For this review, use the dimensioned drawing (mm, ordinates from the lowest corner) and the shaded views. A direction names the side the tool comes from. Give positions to 0.01 mm unless a question says otherwise; leave off trailing zeros. Write each loop counter-clockwise with the first axis right and the second up, starting at its lowest first coordinate (ties: lowest second). Pieces come first, ordered by that corner, then holes. Notation, with made-up numbers: M 42,47.5 L 85,47.5 A23 ccw 85,59.5 Z; hole C 38,65 d7. An arc over 180 degrees is marked long. One line per item, written item: value. Start each with the question number.
Item 1: Consider section C-C, the plane z = 11. Write out the cut boundary in (x, y).
Item 2: Consider section D-D, the plane x = 9. Write out the cut boundary in (y, z), and give its area (3 significant figures).
Item 3: Tool access review of the marked faces 1, 2 and 3: name each direction out of +Z, -Z, +X, -X, +Y, -Y from which nothing blocks a thin tool from reaching the whole face with its end or side.
Item 4: To check wall thickness, follow probe 1 along X at (y, z) = (6.25, 4.75); probe 2 along X at (y, z) = (1.75, 18.5); probe 3 along Z at (x, y) = (25, 14.25). State the ranges of each line that lie inside material, in increasing order.
Item 5: Consider section A-A, the plane z = 5.25. Write out the cut boundary in (x, y).
Item 6: Mouldability with a two-part tool opening along X and no side actions: class the marked faces 4, 5, 6 and 7 as released by +X, released by -X, zero draft, split by the parting line, or undercut.
Item 7: Clearance check with flat-ended pins moving along their axes: pin 1 Ø8 at (y, z) = (7, 4) entering from +X; pin 2 Ø2 at (y, z) = (10, 5) entering from -X; pin 3 Ø4.5 at (x, y) = (20, 10) entering from +Z. State where each tip first meets the part, or that it passes through.
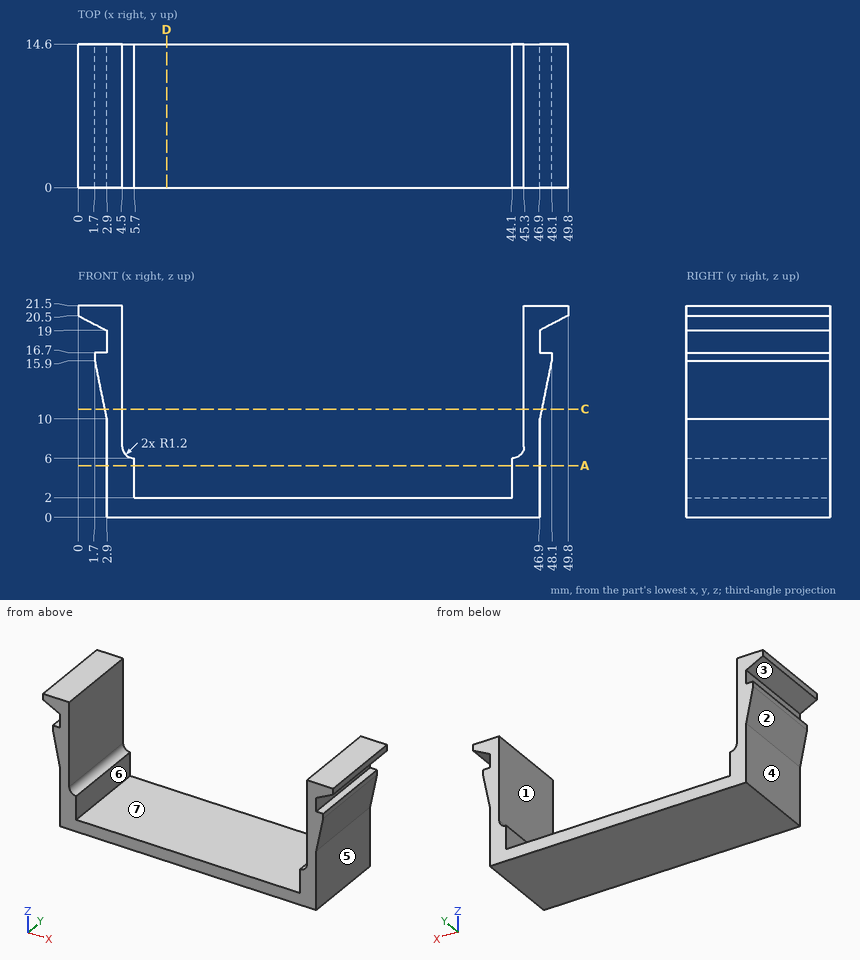
Model answer:
1. outline: M 2.7,0 L 4.5,0 L 4.5,14.6 L 2.7,14.6 Z; M 45.3,0 L 47.1,0 L 47.1,14.6 L 45.3,14.6 Z
2. outline: M 0,0 L 14.6,0 L 14.6,2 L 0,2 Z
2. area: 29.2 mm2
3. face 1: +Z, +Y, -Y
3. face 2: -Z, -X, +Y, -Y
3. face 3: -X, +Y, -Y
4. probe 1: x = 2.9 to 5.7, 44.1 to 46.9
4. probe 2: x = 2.9 to 4.5, 45.3 to 46.9
4. probe 3: z = 0 to 2
5. outline: M 2.9,0 L 5.7,0 L 5.7,14.6 L 2.9,14.6 Z; M 44.1,0 L 46.9,0 L 46.9,14.6 L 44.1,14.6 Z
6. face 4: released by -X
6. face 5: released by +X
6. face 6: undercut
6. face 7: undercut
7. pin 1: stops at x = 46.9
7. pin 2: stops at x = 2.9
7. pin 3: stops at z = 2
